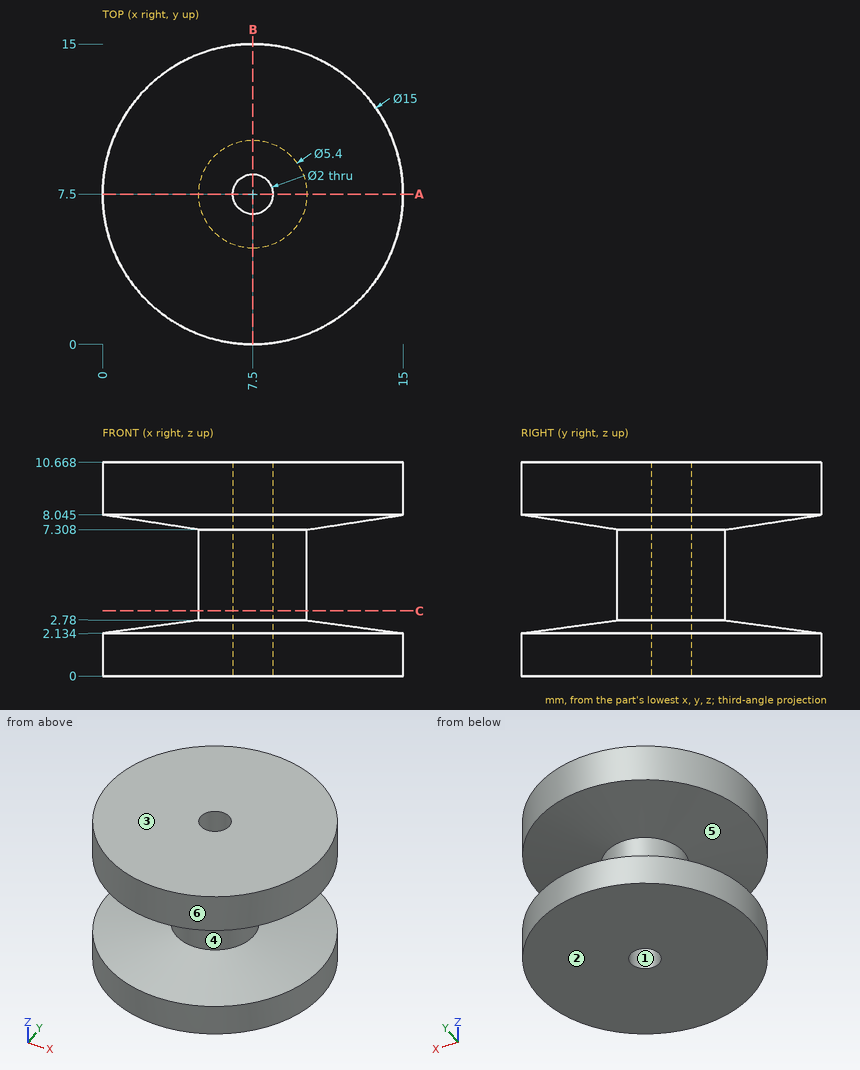
Check sheet for the drawn part. Datum: minimum x, y, z corner. Units: mm. A direction names the side the tool comes from. Round coordinates to 2 decimals unless told otherwise and drop trailing zeros. Loops run counter-clockwise (first coordinate to the right, second up) from the corner with the lowest first, then second, coordinate; pieces in that order, holes last.
Item 1: Access from +Z, -Z, +X, -X, +Y, -Y to the whole of each face (thin tool, end or side, straight path). Record for the marked faces 5 and 6.
Item 2: Cross-section at C-C on z = 3.25. Record the boundary of the cut face in (x, y).
Item 3: Thickness scan on line 1 (Y direction, x = 7.5, z = 5.5); line 2 (Z direction, x = 4, y = 3); line 3 (Z direction, x = 12.75, y = 8) (1 decimal). Record the ranges inside material, lowest first.
Item 4: Cross-section at A-A on y = 7.5. Record the boundary of the cut face in (x, z) (1 decimal).
Item 5: Gauge pin test, flat ends, axial feed: pin 1 (1.5 mm diameter, centred on y = 6, z = 2.5, fed in from -X); pin 2 (1 mm diameter, centred on x = 5, z = 3.5, fed in from +Y) (1 decimal); pin 3 (1 mm diameter, centred on x = 10.5, z = 1, fed in from -Y). Record the tip position at first contact, or that the pin passes through.
Item 6: Mould release check, pull along Z, two halves, no side actions. Record for the marked faces 1, 2, 3 and 4: pulls with the +Z half, pulls with the -Z half, needs draft (parallel to the pull), parting line crosses it, or undercut.
Answer sheet:
1. face 5: none
1. face 6: +Z, -Z
2. outline: circle Ø5.4 at (7.5, 7.5); hole circle Ø2 at (7.5, 7.5)
3. line 1: y = 4.8 to 6.5, 8.5 to 10.2
3. line 2: z = 0 to 2.38, 7.77 to 10.67
3. line 3: z = 0 to 2.4, 7.7 to 10.7
4. outline: (0, 0) - (6.5, 0) - (6.5, 10.7) - (0, 10.7) - (0, 8) - (4.8, 7.3) - (4.8, 2.8) - (0, 2.1) - close; (8.5, 0) - (15, 0) - (15, 2.1) - (10.2, 2.8) - (10.2, 7.3) - (15, 8) - (15, 10.7) - (8.5, 10.7) - close
5. pin 1: stops at x = 0.05
5. pin 2: stops at y = 9.3
5. pin 3: stops at y = 0.43
6. face 1: needs draft
6. face 2: pulls with the -Z half
6. face 3: pulls with the +Z half
6. face 4: undercut
